Model file for the job. Use its own axes, mm. A direction names the side the tool comes from. Give positions to 0.01 mm unless a question says otherwise; leave off trailing zeros. Order: outer loops, then holes, each group sorted by start corner. A loop starts at its lowest first (then second) coordinate and runs counter-clockwise, first axis right, second up. Notation, with made-up numbers: (15, 39) - (42, 39) arc R27 ccw to (42, 55) - close; hole circle Ø6 at (15, 65.5). An arc over 180 degrees is marked (long way). Use CSV: the item, a comma, the result in double quotes. Start each with the question number.
(1) Tool access for faces 5 (the flat face through (-12.5, -16, 0)), 6 (the flat face through (-2, 2.5, 1)), 7 (the flat face through (12.5, -16, 0)), 8 (the flat face through (-12.5, 1, 0)), 9 (the flat face through (5.55, 4, -6)): list every direction of +Z, -Z, +X, -X, +Y, -Y with a clear straight run to the whole face (end or side of a thin tool).
(2) Band-saw the part on A-A, the plane x = 10. Give the cut face in (y, z).
(3) Band-saw the part on B-B, the plane z = -3.25. Count the separate pieces of the cut face and the enclosed holes in it, then the cut area to 3 significant figures.
(4) Band-saw the part on C-C, the plane x = 0. Give the cut face in (y, z).
(5) Band-saw the part on D-D, the plane z = 8.25. Give the cut face in (x, y), then the cut area to 3 significant figures.
(6) Drop flat-ended pins along their axis: pin 1 Ø1.2 at (y, z) = (1.5, -5.5) entering from +X; pin 2 Ø3 at (y, z) = (1, -6) entering from -X; pin 3 Ø3 at (x, y) = (2.5, 4.5) entering from -Z. Give the stop position or say it passes through.
(7) Probe L1, parallel to Y at x = -10, z = 6.5; L2, parallel to X at y = 3.5, z = -5; L3, parallel to Y at x = -1.5, z = 1.75. List the from-to ranges inside material, lowest first.
(8) Pull direction X, two halves, no side cores. Call faces 1 (the flat face through (13, -26, 0)), 2 (the flat face through (0, -30, 0)), 3 (the flat face through (0.55, 4, 3)), 4 (the flat face through (-3, 4, 0.5)): +X half, -X half, draft (parallel to the pull), parting line (faces both ways), or undercut.
from build123d import *

# Parameters (mm, degrees)
F0_W      = 25
F0_H      = 25
F1_DEPTH  = 30
F2_W      = 25
F2_H      = 25
F3_DEPTH  = 5
F5_DEPTH  = 2.5
F7_DEPTH  = 25
F9_W      = 13
F9_H      = 5.4
F10_DEPTH = 12.5
F8_R      = 2.15
F11_DEPTH = 12.5


with BuildPart() as f1:
    # F0 (on Front) → F1 (new body)
    with BuildSketch(Plane.XZ):
        Rectangle(F0_W, F0_H)
    extrude(amount=F1_DEPTH)

    # F2 (on Front) → F3 (join)
    with BuildSketch(Plane.XZ):
        Rectangle(F2_W, F2_H)
    extrude(amount=-F3_DEPTH)

    # F4 (on Front) → F5 (cut)
    with BuildSketch(Plane.XZ):
        with BuildLine():
            ThreePointArc((-9, 0), (0, -9), (9, 0))
            ThreePointArc((9, 0), (0, 9), (-9, 0))
        make_face()
        with BuildLine():
            Line((9, -12.5), (9, 0))
            ThreePointArc((9, 0), (0, -9), (-9, 0))
            Line((-9, 0), (-9, -12.5))
            Line((-9, -12.5), (9, -12.5))
        make_face()
    extrude(amount=-F5_DEPTH, mode=Mode.SUBTRACT)

    # F6 (on Front) → F7 (cut)
    with BuildSketch(Plane.XZ):
        Polygon((0.55, 0.5), (0.55, 5.3), (-0.55, 5.3), (-0.55, 0.5), (-5.55, 0.5), (-5.55, -12.5), (5.55, -12.5), (5.55, 0.5), align=None)
    extrude(amount=-F7_DEPTH, mode=Mode.SUBTRACT)

    # F9 (on Top) → F10 (join, symmetric)
    with BuildSketch(Plane.XY):
        with Locations((-6.5, -6)):
            Rectangle(F9_W, F9_H)
        with Locations((6.5, -6)):
            Rectangle(F9_W, F9_H)
        with Locations((-6.5, -26)):
            Rectangle(F9_W, F9_H)
        with Locations((6.5, -26)):
            Rectangle(F9_W, F9_H)
    extrude(amount=F10_DEPTH, both=True)

    # F8 (on Top) → F11 (cut, symmetric)
    with BuildSketch(Plane.XY):
        with Locations((-10, -6)):
            Circle(F8_R)
        with Locations((-10, -26)):
            Circle(F8_R)
        with Locations((10, -6)):
            Circle(F8_R)
        with Locations((10, -26)):
            Circle(F8_R)
    extrude(amount=F11_DEPTH, both=True, mode=Mode.SUBTRACT)


solid = f1.part
Answer block:
1,face 5,"+Z, -Z, -X"
1,face 6,"-Z"
1,face 7,"+Z, -Z, +X"
1,face 8,"+Z, -Z, -X, +Y"
1,face 9,"-Z, +Y"
2,outline,"(-30, -12.5) - (-28.15, -12.5) - (-28.15, 12.5) - (-30, 12.5) - close; (-23.85, -12.5) - (-8.15, -12.5) - (-8.15, 12.5) - (-23.85, 12.5) - close; (-3.85, -12.5) - (5, -12.5) - (5, 12.5) - (-3.85, 12.5) - close"
3,separate pieces,"1"
3,enclosed holes,"4"
3,area,"755 mm2"
4,outline,"(-30, -12.5) - (0, -12.5) - (0, 9) - (2.5, 9) - (2.5, 5.3) - (5, 5.3) - (5, 12.5) - (-30, 12.5) - close"
5,outline,"(-13, -28.7) - (-12.5, -28.7) - (-12.5, -30) - (12.5, -30) - (12.5, -28.7) - (13, -28.7) - (13, -23.3) - (12.5, -23.3) - (12.5, -8.7) - (13, -8.7) - (13, -3.3) - (12.5, -3.3) - (12.5, 5) - (-12.5, 5) - (-12.5, -3.3) - (-13, -3.3) - (-13, -8.7) - (-12.5, -8.7) - (-12.5, -23.3) - (-13, -23.3) - close; hole circle Ø4.3 at (-10, -26); hole circle Ø4.3 at (-10, -6); hole (-3.6, 0) - (3.6, 0) - (3.6, 2.5) - (-3.6, 2.5) - close; hole circle Ø4.3 at (10, -26); hole circle Ø4.3 at (10, -6)"
5,area,"810 mm2"
6,pin 1,"stops at x = 12.5"
6,pin 2,"stops at x = -12.5"
6,pin 3,"stops at z = 0.5"
7,L1,"y = -30 to -28.15, -23.85 to -8.15, -3.85 to 5"
7,L2,"x = -12.5 to -5.55, 5.55 to 12.5"
7,L3,"y = -30 to 0, 2.5 to 5"
8,face 1,"+X half"
8,face 2,"draft"
8,face 3,"undercut"
8,face 4,"undercut"
